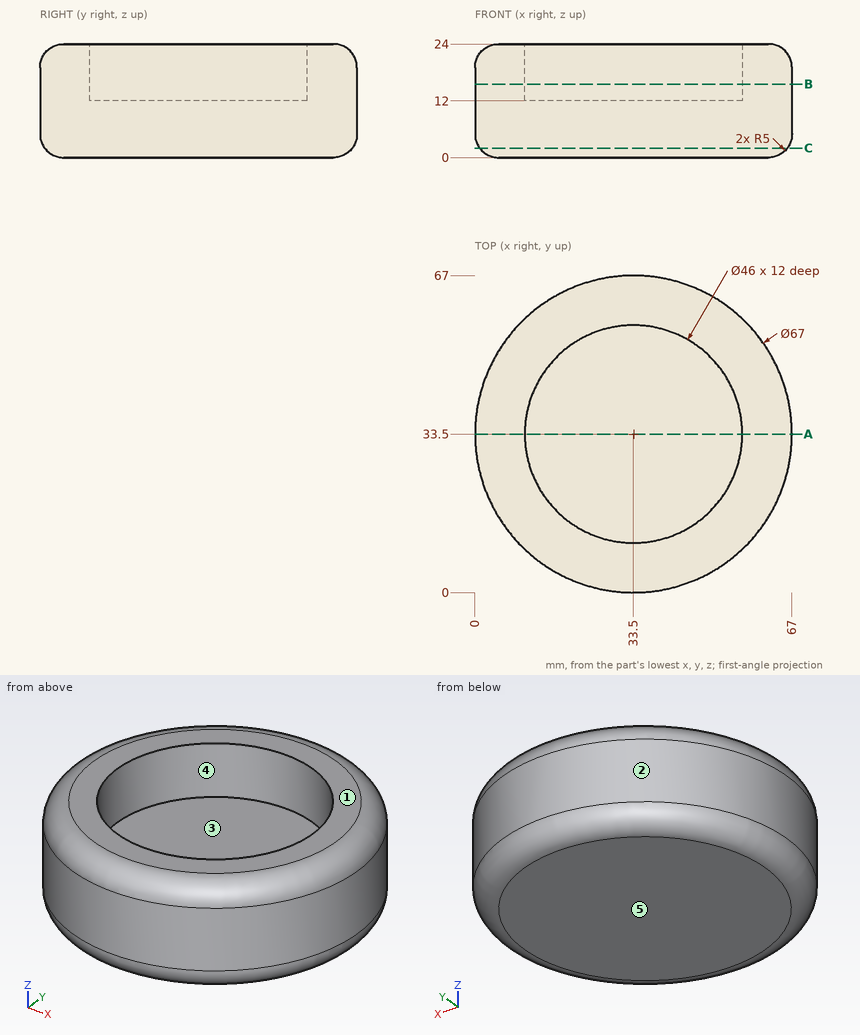
Check sheet for the drawn part. Datum: minimum x, y, z corner. Units: mm. A direction names the side the tool comes from. Round coordinates to 2 decimals unless told otherwise and drop trailing zeros. Order: outer loops, then holes, each group sorted by start corner. A loop starts at its lowest first (then second) coordinate and runs counter-clockwise, first axis right, second up. Notation, with made-up numbers: (55.5, 74.25) -> (94.5, 74.25) arc R18 ccw to (94.5, 80.25) -> close; hole circle Ø1 at (6.5, -24). An arc over 180 degrees is marked (long way). Use CSV: the item, a comma, the result in double quotes.
(1) Cross-section at A-A (y = 33.5). Record the boundary of the cut face in (x, z), and give its area (3 significant figures).
Worked out:
outline,"(0, 5) arc R5 ccw to (5, 0) -> (62, 0) arc R5 ccw to (67, 5) -> (67, 19) arc R5 ccw to (62, 24) -> (56.5, 24) -> (56.5, 12) -> (10.5, 12) -> (10.5, 24) -> (5, 24) arc R5 ccw to (0, 19) -> close"
area,"1,030 mm²"
(2) Depth check by flat-ended pin: pin 1 (12 mm diameter, centred on y = 58, z = 13.5, fed in from -X); pin 2 (6 mm diameter, centred on y = 48, z = 14, fed in from -X); pin 3 (8 mm diameter, centred on y = 59.5, z = 4, fed in from +X). Enter the tip coordinate at first touch or a pass-through.
Worked out:
pin 1,"x = 5.57"
pin 2,"x = 2.04"
pin 3,"x = 58.7"
(3) Cross-section at B-B (z = 15.5). Record the boundary of the cut face in (x, y), and give its area (3 significant figures).
Worked out:
outline,"circle Ø67 at (33.5, 33.5); hole circle Ø46 at (33.5, 33.5)"
area,"1,860 mm²"
(4) Material ranges on line 1 along Y through (x, z) = (33.5, 18); line 2 along Z through (x, y) = (47.5, 22.5); line 3 along Y through (x, z) = (40, 12.25), recorded low to high. Write a range as from..to.
Worked out:
line 1,"0..10.5, 56.5..67"
line 2,"0..12"
line 3,"0.64..11.44, 55.56..66.36"
(5) Draft check along X on the marked faces 1, 2 and 3. Enter one of: pulls with the +X half, pulls with the -X half, needs draft (parallel to the pull), parting line crosses it, or undercut.
Worked out:
face 1,"needs draft"
face 2,"parting line crosses it"
face 3,"undercut"
(6) Tool access check on the marked faces 4 and 5. Record the directions out of +Z, -Z, +X, -X, +Y, -Y that give a thin tool (end or side, any length) a straight path to the whole face; none if there is none.
Worked out:
face 4,"+Z"
face 5,"-Z, +X, -X, +Y, -Y"
(7) Cross-section at C-C (z = 2). Record the boundary of the cut face in (x, y).
Worked out:
outline,"circle Ø65 at (33.5, 33.5)"
